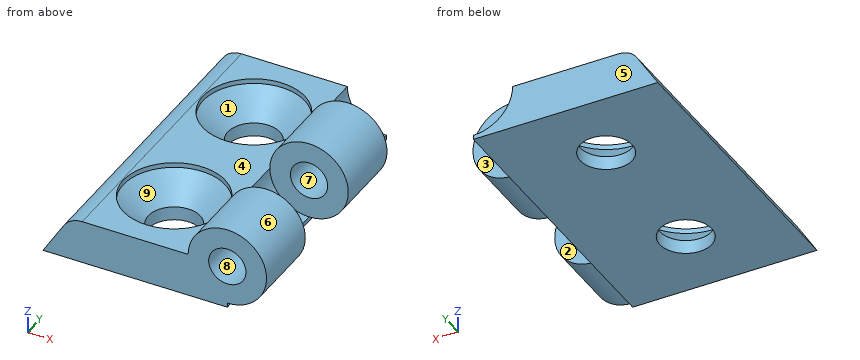
```python
from build123d import *

# Parameters (mm, degrees)
SKETCH1_R                                    = 1.9
BOSS_EXTRUDE1_DEPTH                          = 7.3
BOSS_EXTRUDE2_DEPTH                          = 30
BOSS_EXTRUDE5_START                          = 15.4
SKETCH1_7_R                                  = 4
SKETCH1_7_R_2                                = 1.9
BOSS_EXTRUDE5_DEPTH                          = 7.3
CSK_FOR_M5_COUNTERSUNK_FLAT_HEAD_SCR_2_COUNT = 2
CSK_FOR_M5_COUNTERSUNK_FLAT_HEAD_SCR_2_PITCH = 15


with BuildPart() as part:
    # Sketch1 → Boss-Extrude1 (new body)
    with BuildSketch(Plane(origin=(0, 0, 0), x_dir=(1, 0, 0), z_dir=(0, 1, 0))):
        with BuildLine():
            Line((0, 4), (0, 4.45))
            Line((0, 4.45), (-18.8, 4.45))
            Line((-18.8, 4.45), (-16.690397065, 1.051533367))
            ThreePointArc((-16.690397065, 1.051533367), (-15.8815872, 0.280573573), (-14.8, 0))
            Line((-14.8, 0), (-4, 0))
            ThreePointArc((-4, 0), (2.828427125, -2.828427125), (0, 4))
        make_face()
        Circle(SKETCH1_R, mode=Mode.SUBTRACT)
    extrude(amount=BOSS_EXTRUDE1_DEPTH)

    # Sketch1_3 → Boss-Extrude2 (add)
    with BuildSketch(Plane(origin=(0, 0, 0), x_dir=(1, 0, 0), z_dir=(0, 1, 0))):
        with BuildLine():
            Line((0, 4), (0, 4.45))
            Line((0, 4.45), (-18.8, 4.45))
            Line((-18.8, 4.45), (-16.690397065, 1.051533367))
            ThreePointArc((-16.690397065, 1.051533367), (-15.8815872, 0.280573573), (-14.8, 0))
            Line((-14.8, 0), (-4, 0))
            ThreePointArc((-4, 0), (-2.828427125, 2.828427125), (0, 4))
        make_face()
    extrude(amount=BOSS_EXTRUDE2_DEPTH)

    # Sketch1_7 → Boss-Extrude5 (add)
    with BuildSketch(Plane(origin=(0, 0, 0), x_dir=(1, 0, 0), z_dir=(0, 1, 0)).offset(BOSS_EXTRUDE5_START)):
        Circle(SKETCH1_7_R)
        Circle(SKETCH1_7_R_2, mode=Mode.SUBTRACT)
    extrude(amount=BOSS_EXTRUDE5_DEPTH)

    # Sketch3 → CSK for M5 Countersunk Flat Head Screw1 (revolve, cut)
    with BuildSketch(Plane(origin=(-9.475, 22.5, 0), x_dir=(0, -1, 0), z_dir=(1, 0, 0))):
        Polygon((0, 0), (0, 4.45), (2.65, 4.45), (2.65, 3.05), (5.2, 0.5), (5.2, 0), align=None)
    csk_for_m5_countersunk_flat_head_screw1 = revolve(axis=Axis((-9.475, 22.5, 6.35), (0, 0, -1)), mode=Mode.SUBTRACT)

    # CSK for M5 Countersunk Flat Head Scr 2: CSK for M5 Countersunk Flat Head Screw1 ×2
    with Locations(*[(0, -i * CSK_FOR_M5_COUNTERSUNK_FLAT_HEAD_SCR_2_PITCH, 0) for i in range(1, CSK_FOR_M5_COUNTERSUNK_FLAT_HEAD_SCR_2_COUNT)]):
        add(csk_for_m5_countersunk_flat_head_screw1, mode=Mode.SUBTRACT)


solid = part.part
```
The listing builds one solid part. Answer for the finished solid, in the listing's coordinates (mm). Face numbers are marked on the shaded views. A direction names the side the tool comes from. Give positions to 0.01 mm unless a question says otherwise; leave off trailing zeros. Order: outer loops, then holes, each group sorted by start corner. A loop starts at its lowest first (then second) coordinate and runs counter-clockwise, first axis right, second up. Notation, with made-up numbers: M 1.5,-14.5 L 10.5,-14.5 A24 cw 10.5,0.5 Z; hole C -20.5,67.5 d6. An arc over 180 degrees is marked long. Put each result on its own line as item: value. Start each with the question number.
Item 1: For a pull along Z with two mould halves and no side action, classify the marked faces 6, 7, 8 and 9 as +Z half, -Z half, draft (parallel to the pull), parting line (faces both ways), or undercut.
Item 2: Flat-ended cylindrical pins translate along their axes: P1, Ø2.5, axis at x = 0, z = 0, coming from the -Y side; P2, Ø8.5, axis at x = -11, y = 22, coming from the +Z side; P3, Ø2, axis at y = 16.5, z = 2.5, coming from the +X side; P4, Ø3, axis at y = 25.5, z = 0, coming from the +X side. Find the tip coordinate at first contact, or state that the pin passes through.
Item 3: The part is cut by section C-C, the plane y = 6. State how many separate pieces and enclosed holes the cut face has, and give its area (3 significant figures).
Item 4: The part is cut by section B-B, the plane x = -2.25. Determine the outline of the cut face in (y, z), and give its area (3 significant figures).
Item 5: The part is cut by section A-A, the plane y = 14.25. Determine the outline of the cut face in (x, z) (3 decimals).
Item 6: Which of the six approach directions +Z, -Z, +X, -X, +Y, -Y give full straight-line access (tool end or side, diameter ignored) to the marked faces 1, 2, 3, 4 and 5?
Item 7: Find the intervals of material crossed by line 1 along Y through (x, z) = (-1, -3.75); line 2 along Y through (x, z) = (-11, -0.25); line 3 along X through (y, z) = (10.5, -1.25), in increasing order.
Answer key:
1. face 6: parting line
1. face 7: undercut
1. face 8: undercut
1. face 9: +Z half
2. P1: passes through
2. P2: stops at z = 0
2. P3: stops at x = 3.71
2. P4: stops at x = -3.71
3. separate pieces: 2
3. enclosed holes: 1
3. area: 74.1 mm²
4. outline: M 0,-4.45 L 30,-4.45 L 30,-3.31 L 22.7,-3.31 L 22.7,3.31 L 15.4,3.31 L 15.4,-3.31 L 7.3,-3.31 L 7.3,3.31 L 0,3.31 Z
4. area: 131 mm²
5. outline: M -18.8,-4.45 L 0,-4.45 L 0,-4 A4 cw -4,0 L -14.8,0 A2.225 ccw -16.69,-1.052 Z
6. face 1: +Z
6. face 2: +Z, +X
6. face 3: +Z, +X, +Y
6. face 4: +Z, -X, +Y, -Y
6. face 5: +Z, -Z, +X, -X, +Y
7. line 1: y = 0 to 7.3, 15.4 to 22.7
7. line 2: y = 0 to 2.53, 12.47 to 17.53, 27.47 to 30
7. line 3: x = -16.81 to -12.76, -6.19 to -3.8
